Autodesk Inventor part; units mm, degrees
ref_plane "YZ Plane" through (0, 0, 0) normal (1, 0, 0) x (0, 1, 0)
ref_plane "XZ Plane" through (0, 0, 0) normal (0, 1, 0) x (-1, 0, 0)
ref_plane "XY Plane" through (0, 0, 0) normal (0, 0, 1) x (1, 0, 0)
sketch "Skizze1" plane through (0, 0, 0) normal (0, 1, 0) x (-1, 0, 0)
  point P0 (0, 0)
sketch "Skizze2" plane through (0, 0, 0) normal (1, 0, 0) x (0, 1, 0)
  line L0 (5, 0) -> (17, 0)
  line L1 (17, -13) -> (0, -13)
  line L2 (0, -13) -> (0, -5)
  line L3 (5, 0) -> (0, -5)
  line L4 (17, -3) -> (6, -3)
  line L5 (6, -3) -> (6, -9)
  line L6 (6, -9) -> (17, -9)
  line L7 (17, 0) -> (17, -3)
  line L8 (17, -9) -> (17, -13)
  point P0 (0, 0)
  point P1 (17, -11)
  dimension "d1" = 13
  dimension "d2" = 5
  dimension "d5" = 3
  dimension "d6" = 4
  dimension "d7" = 11
  dimension "d8" = 12
  dimension "d9" = 17
extrude "Extrusion1" add sketch "Skizze2" along normal mid plane 10
fillet "Rundung1" radius 5 2 edges at (5, 17, -1.5) (-5, 17, -1.5)
fillet "Rundung2" radius 5 2 edges at (5, 17, -11) (-5, 17, -11)
sketch "Skizze4" plane through (5, 0, -13) normal (0, 0, -1) x (-1, 0, 0)
  arc A0 (10, 12) -> (0, 12) centre (5, 12) ccw
  point P0 (5, 0)
hole "Bohrung1" at (0, 12, -13) direction (0, 0, 1) diameter 4.134 depth 4
sketch "Skizze5" plane through (-5, 5, 0) normal (0, 0, 1) x (1, 0, 0)
  arc A0 (10, 7) -> (0, 7) centre (5, 7) ccw
  point P0 (5, -5)
hole "Bohrung2" at (0, 12, 0) direction (0, 0, -1) diameter 4.134 depth 3
sketch "Skizze6" plane through (5, 0, -13) normal (0, 0, -1) x (-1, 0, 0)
  line L0 (0, 0) -> (-1, -109)
  line L1 (10, 0) -> (0, 0)
  line L2 (10, 0) -> (11, -109)
  line L3 (5, 0) -> (5, -23.6685) construction
  line L4 (-1, -109) -> (11, -109)
  circle A0 centre (5, 12) radius 2.067
  dimension "d29" = 12
  dimension "d30" = 121
extrude "Extrusion2" add sketch "Skizze6" against normal blind 4 contours L1 L2 L4 L0
fillet "Rundung3" radius 2 2 edges at (0, 0, -5) (0, 5, 0)
sketch "Skizze7" plane through (0, 12, -13) normal (0, 0, -1) x (-1, 0, 0)
  line L0 (-14, -121) -> (14, -121)
  line L1 (14, -121) -> (14, -124)
  line L2 (14, -124) -> (-14, -124)
  line L3 (-14, -124) -> (-14, -121)
  line L4 (-6, -121) -> (6, -121)
  point P0 (0, -12)
  point P1 (0, -124)
  point P2 (0, -121)
  point P3 (0, -121)
  dimension "d34" = 28
  dimension "d35" = 3
extrude "Extrusion3" add sketch "Skizze7" against normal blind 10
fillet "Rundung4" radius 0.5 3 edges at (6, -109, -11) (-6, -109, -11) (0, -109, -9)
sketch "Skizze8" plane through (-14, -109, -3) normal (0, 1, 0) x (1, 0, 0)
  line L0 (9, 10) -> (19, 10)
  line L1 (0, 10) -> (0, 0)
  point P0 (14, -3)
  point P1 (4, 5)
  point P2 (24, 5)
  point P3 (14, 10)
  point P4 (14, 10)
  point P5 (0, 5)
  dimension "d46" = 10
  dimension "d47" = 10
hole "Bohrung3" at (-10, -109, -8) at (10, -109, -8) direction (0, -1, 0) diameter 4 depth 3
properties part number "205" material "Aluminium 6061"
Could you check a few things on this model? Use its own coordinates, in mm. A direction names the side the tool comes from. Round coordinates to 2 decimals unless told otherwise and drop trailing zeros. Order: outer loops, then holes, each group sorted by start corner. A loop starts at its lowest first (then second) coordinate and runs counter-clockwise, first axis right, second up. Notation, with made-up numbers: M -5,44.5 L 43,44.5 A32 cw 43,81.5 Z; hole C -9.75,-4.5 d10. An arc over 180 degrees is marked long. One line per question, with ' | ' between items. Start each with the question number.
(1) For P1, Ø6, axis at x = 1.5, y = -46, coming from the +Z side; P2, Ø2.5, axis at x = 4.5, y = -110, coming from the +Z side; P3, Ø5, axis at y = -87.5, z = -8, coming from the +X side, each with a flat end and sliding along its axis, tell me the tip position at first contact or that it passes through.
(2) For faces 1 (the face through (1, 10, -9)), 2 (the face through (0, 3, -2)), 3 (the face through (0, -109, -7)), 4 (the face through (-4, 15, -2)), which set-ups out of +Z, -Z, +X, -X, +Y, -Y let a thin tool reach every point of the face, with its end or its side?
(3) Suppose I cut it at A-A on x = 10. List the corners of the cut face in (y, z) for me, then the cut area to 3 significant figures.
(4) Thinking about a two-plate mould opening in X: for faces 5 (the face through (5, 5, -6)), 6 (the face through (-5, 5, -6)), 7 (the face through (-0.091, 14.065, -1.521)), which applies, +X half, -X half, draft (parallel to the pull), parting line (faces both ways), or undercut?
(5) Please list where these lines run through material, in increasing order: line 1 along X through (y, z) = (-111.3, -8); line 2 along Y through (x, z) = (1, -6.75); line 3 along X through (y, z) = (12, -11.35).
Geometry results:
1) P1: z = -9 | P2: z = -3 | P3: x = 5.82
2) face 1: +X, -X, +Y | face 2: +Z, +X, -X | face 3: +Z | face 4: +Z, -Z, -X, +Y
3) outline: M -112,-13 L -109,-13 L -109,-10 L -112,-10 Z; M -112,-6 L -109,-6 L -109,-3 L -112,-3 Z | area: 18.0 mm²
4) face 5: +X half | face 6: -X half | face 7: undercut
5) line 1: -14 to -12, -8 to 8, 12 to 14 | line 2: -112 to -109, 0 to 6 | line 3: -5 to -2.07, 2.07 to 5
